from build123d import *

# Parameters (mm, degrees)
ESQUISSE1_R        = 3.2
ESQUISSE1_R_2      = 15
BOSS_EXTRU_1_DEPTH = 5


with BuildPart() as part:
    # Esquisse1 → Boss.-Extru.1 (new body)
    with BuildSketch(Plane(origin=(0, 0, 0), x_dir=(1, 0, 0), z_dir=(0, 1, 0))):
        with BuildLine():
            Line((95.704424879, -12.251847565), (76.653223752, -1.249496196))
            Line((76.653223752, -1.249496196), (87.655575121, 17.80170493))
            Line((87.655575121, 17.80170493), (94.826792906, 30.219078976))
            ThreePointArc((94.826792906, 30.219078976), (83.075750919, 47.929028471), (73.600020266, 66.953744698))
            Line((73.600020266, 66.953744698), (59.253871219, 66.953744698))
            Line((59.253871219, 66.953744698), (37.253871219, 66.953744698))
            Line((37.253871219, 66.953744698), (37.253871219, 88.953744698))
            Line((37.253871219, 88.953744698), (59.253871219, 88.953744698))
            Line((59.253871219, 88.953744698), (66.003069732, 88.953744698))
            ThreePointArc((66.003069732, 88.953744698), (61.294306765, 112.991978793), (60.05, 137.455438234))
            ThreePointArc((60.05, 137.455438234), (0, 150), (-60.05, 137.455438234))
            ThreePointArc((-60.05, 137.455438234), (-61.294306765, 112.991978793), (-66.003069732, 88.953744698))
            Line((-66.003069732, 88.953744698), (-59.253871219, 88.953744698))
            Line((-59.253871219, 88.953744698), (-37.253871219, 88.953744698))
            Line((-37.253871219, 88.953744698), (-37.253871219, 66.953744698))
            Line((-37.253871219, 66.953744698), (-59.253871219, 66.953744698))
            Line((-59.253871219, 66.953744698), (-73.600020266, 66.953744698))
            ThreePointArc((-73.600020266, 66.953744698), (-83.054066993, 47.966565203), (-94.774500839, 30.288233406))
            Line((-94.774500839, 30.288233406), (-87.606022607, 17.864984041))
            Line((-87.606022607, 17.864984041), (-76.610725847, -1.190289486))
            Line((-76.610725847, -1.190289486), (-95.665999373, -12.185586245))
            Line((-95.665999373, -12.185586245), (-106.661296133, 6.869687281))
            Line((-106.661296133, 6.869687281), (-110.03272827, 12.712509258))
            ThreePointArc((-110.03272827, 12.712509258), (-128.500854083, -3.381043685), (-149.069024712, -16.686098152))
            ThreePointArc((-149.069024712, -16.686098152), (-129.922319498, -74.967932452), (-89.044700128, -120.710568631))
            ThreePointArc((-89.044700128, -120.710568631), (-67.232592853, -109.561304368), (-44.057183789, -101.625654924))
            Line((-44.057183789, -101.625654924), (-47.428615926, -95.782832947))
            Line((-47.428615926, -95.782832947), (-58.423912686, -76.727559421))
            Line((-58.423912686, -76.727559421), (-39.36863916, -65.732262661))
            Line((-39.36863916, -65.732262661), (-28.3733424, -84.787536188))
            Line((-28.3733424, -84.787536188), (-21.204864167, -97.210785553))
            ThreePointArc((-21.204864167, -97.210785553), (0.007838221, -95.910230344), (21.218905144, -97.237191709))
            Line((21.218905144, -97.237191709), (28.390122928, -84.819817663))
            Line((28.390122928, -84.819817663), (39.392474297, -65.768616537))
            Line((39.392474297, -65.768616537), (58.443675423, -76.770967905))
            Line((58.443675423, -76.770967905), (47.441324055, -95.822169032))
            Line((47.441324055, -95.822169032), (44.059067466, -101.678739902))
            ThreePointArc((44.059067466, -101.678739902), (67.188172186, -109.626679928), (88.955287671, -120.776474511))
            ThreePointArc((88.955287671, -120.776474511), (129.894553134, -75.01603206), (149.069024712, -16.686098152))
            ThreePointArc((149.069024712, -16.686098152), (128.532739261, -3.405050916), (110.089032837, 12.655924432))
            Line((110.089032837, 12.655924432), (106.706776248, 6.799353561))
            Line((106.706776248, 6.799353561), (95.704424879, -12.251847565))
        make_face()
        with Locations(Location((14.5, 76.893024973, 0), (0, 0, 270))):
            Circle(ESQUISSE1_R, mode=Mode.SUBTRACT)
        with Locations(Location((-14.5, 76.893024973, 0), (0, 0, 270))):
            Circle(ESQUISSE1_R, mode=Mode.SUBTRACT)
        with Locations(Location((-73.847701188, -25.870916463, 0), (0, 0, 270))):
            Circle(ESQUISSE1_R, mode=Mode.SUBTRACT)
        with Locations(Location((-59.353900914, -50.989231566, 0), (0, 0, 270))):
            Circle(ESQUISSE1_R, mode=Mode.SUBTRACT)
        with Locations(Location((59.348929552, -51.019238622, 0), (0, 0, 270))):
            Circle(ESQUISSE1_R, mode=Mode.SUBTRACT)
        with Locations(Location((73.852029084, -25.906291683, 0), (0, 0, 270))):
            Circle(ESQUISSE1_R, mode=Mode.SUBTRACT)
        with Locations(Location((0, 0, 0), (0, 0, 270))):
            Circle(ESQUISSE1_R_2, mode=Mode.SUBTRACT)
    extrude(amount=BOSS_EXTRU_1_DEPTH)


solid = part.part
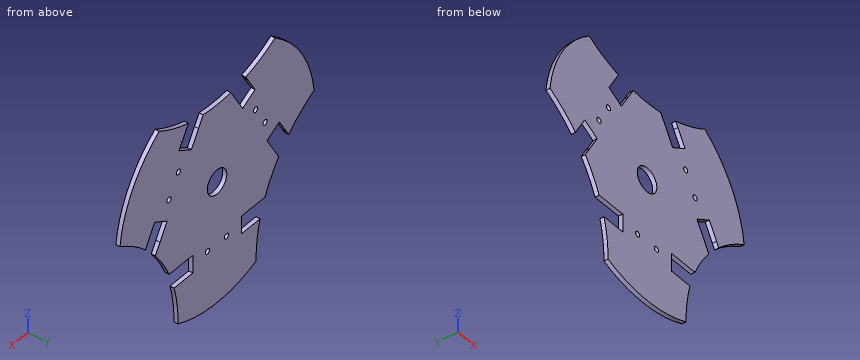
Could you check a few things on this model? Use its own coordinates, in mm. Round coordinates to 2 decimals unless told otherwise and drop trailing zeros. Write each loop counter-clockwise with the first axis right and the second up, starting at its lowest first coordinate (ties: lowest second). Pieces come first, ordered by that corner, then holes. Notation, with made-up numbers: (31.25, 42) -> (68.25, 42) arc R13 ccw to (68.25, 56) -> close; hole circle Ø6 at (31.25, 88.5). An arc over 180 degrees is marked (long way). Use a Markdown table: item, result.
1. Please list where these lines run through material, in increasing order: probe 1 along X at (y, z) = (3.3, 70) (3 decimals); probe 2 along X at (y, z) = (3.55, 0); probe 3 along Z at (x, y) = (-56, 2.95).
Answer key:
| item | result |
|---|---|
| probe 1 | x = -132.665 to -46.765, -36.906 to 36.949, 46.719 to 132.665 |
| probe 2 | x = -124.16 to -102.7, -77.3 to -15, 15 to 77.37, 102.78 to 124.16 |
| probe 3 | z = -139.15 to -88.95, -66.95 to 75.33, 80.93 to 105.25 |
2. If we section it at B-B (x = 0): List the corners of the cut face in (y, z) for me, then the cut area to 3 significant figures.
Answer key:
| item | result |
|---|---|
| outline | (0, -150) -> (5, -150) -> (5, -15) -> (0, -15) -> close; (0, 15) -> (5, 15) -> (5, 95.91) -> (0, 95.91) -> close |
| area | 1,080 mm^2 |
3. If we section it at D-D (z = -62): List the corners of the cut face in (x, y) for me, then the cut area to 3 significant figures.
Answer key:
| item | result |
|---|---|
| outline | (-75.79, 0) -> (75.79, 0) -> (75.79, 5) -> (-75.79, 5) -> close |
| area | 758 mm^2 |
4. If we section it at C-C (y = 2.1): State how many separate pieces and enclosed holes the cut face has, then the cut area to 3 significant figures.
Answer key:
| item | result |
|---|---|
| separate pieces | 1 |
| enclosed holes | 7 |
| area | 45,900 mm^2 |
5. For pin 1 Ø8.5 at (x, z) = (-73.85, 25.87) entering from +Y; pin 2 Ø2.5 at (x, y) = (-44.5, 3.5) entering from +Z; pin 3 Ø1 at (x, y) = (46.5, 3) entering from +Z; pin 4 Ø1.5 at (x, y) = (-10, 1.5) entering from +Z, each with a flat end and sliding along its axis, tell me the tip position at first contact or that it passes through.
Answer key:
| item | result |
|---|---|
| pin 1 | stops at y = 5 |
| pin 2 | stops at z = 102.08 |
| pin 3 | stops at z = 102.49 |
| pin 4 | stops at z = 96.24 |
6. If we section it at A-A (z = 92): List the corners of the cut face in (x, y) for me, then the cut area to 3 significant figures.
Answer key:
| item | result |
|---|---|
| outline | (-118.47, 0) -> (-49.61, 0) -> (-49.61, 5) -> (-118.47, 5) -> close; (-24.21, 0) -> (24.24, 0) -> (24.24, 5) -> (-24.21, 5) -> close; (49.65, 0) -> (118.47, 0) -> (118.47, 5) -> (49.65, 5) -> close |
| area | 931 mm^2 |
